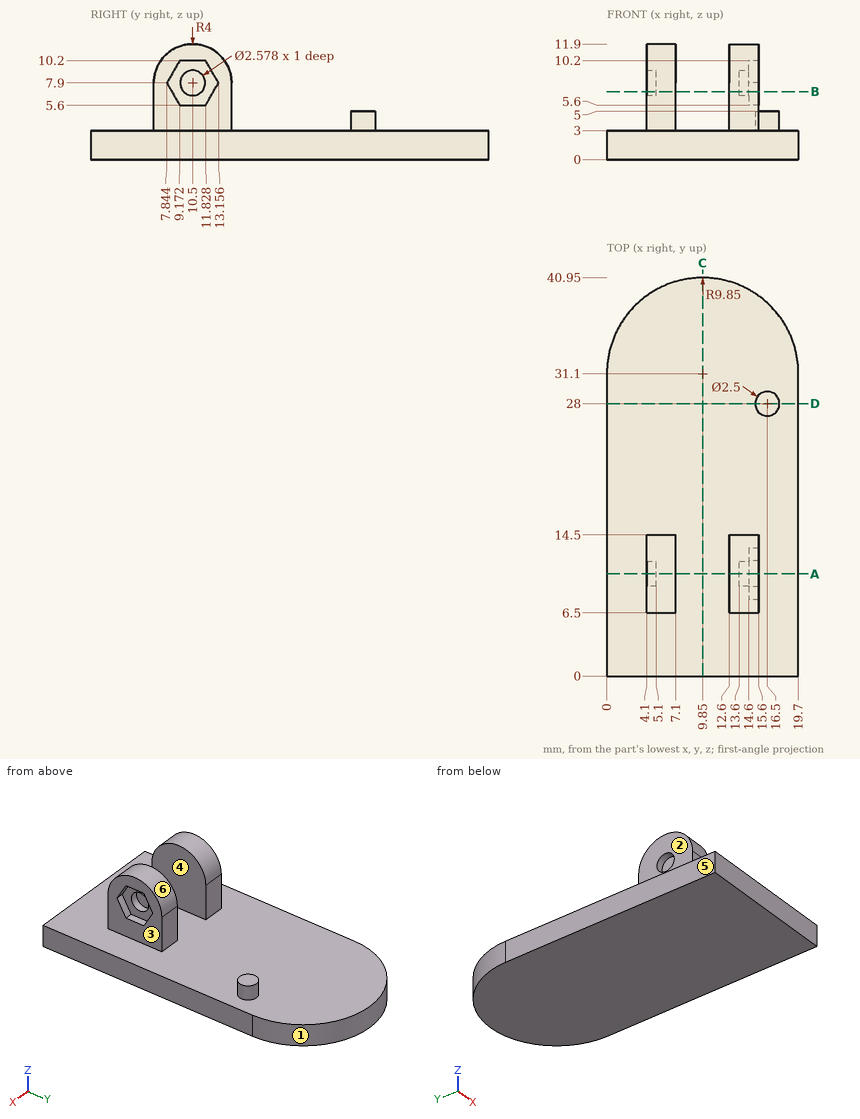
Print and shaded views of the part. All mm, measured from the part's lowest x, y and z. A direction names the side the tool comes from. Round coordinates to 2 decimals unless told otherwise and drop trailing zeros. Write each loop counter-clockwise with the first axis right and the second up, starting at its lowest first coordinate (ties: lowest second). Pieces come first, ordered by that corner, then holes.
(1) Slice it at A-A, the plane y = 10.5. Write the cut outline in (x, z).
(2) Probe line 1 along Z through (x, y) = (14.2, 10.5); line 2 along Y through (x, z) = (4.4, 7.9); line 3 along Z through (x, y) = (2, 26). List the from-to ranges inside material, lowest first.
(3) Mould opens along X. For the marked faces 4, 5 and 6 say: pulls with the +X half, pulls with the -X half, needs draft (parallel to the pull), parting line crosses it, or undercut.
(4) Slice it at D-D, the plane y = 28. Write the cut outline in (x, z), and give its area (3 significant figures).
(5) Drop flat-ended pins along their axis: P1, Ø4, axis at y = 9.5, z = 6, coming from the -X side; P2, Ø2.5, axis at y = 9.5, z = 6, coming from the +X side; P3, Ø1.5, axis at y = 10.5, z = 7.9, coming from the +X side. Give the stop position or say it passes through.
(6) Slice it at B-B, the plane z = 7. Write the cut outline in (x, y).
(7) 3-axis set-ups, long thin cutter, end or side, ignore diameter. For the marked faces 1, 2 and 3: which of +Z, -Z, +X, -X, +Y, -Y reach the whole face in a straight line?
(8) Slice it at C-C, the plane x = 9.85. Write the cut outline in (y, z).
From the geometry:
1. outline: (0, 0) - (19.7, 0) - (19.7, 3) - (15.6, 3) - (15.6, 5.6) - (14.6, 5.6) - (14.6, 6.61) - (13.6, 6.61) - (13.6, 9.19) - (14.6, 9.19) - (14.6, 10.2) - (15.6, 10.2) - (15.6, 11.9) - (12.6, 11.9) - (12.6, 3) - (7.1, 3) - (7.1, 11.9) - (4.1, 11.9) - (4.1, 9.19) - (5.1, 9.19) - (5.1, 6.61) - (4.1, 6.61) - (4.1, 3) - (0, 3) - close
2. line 1: z = 0 to 6.61, 9.19 to 11.9
2. line 2: y = 6.5 to 9.21, 11.79 to 14.5
2. line 3: z = 0 to 3
3. face 4: undercut
3. face 5: pulls with the -X half
3. face 6: needs draft
4. outline: (0, 0) - (19.7, 0) - (19.7, 3) - (17.75, 3) - (17.75, 5) - (15.25, 5) - (15.25, 3) - (0, 3) - close
4. area: 64.1 mm2
5. P1: stops at x = 4.1
5. P2: stops at x = 15.6
5. P3: stops at x = 13.6
6. outline: (4.1, 6.5) - (7.1, 6.5) - (7.1, 14.5) - (4.1, 14.5) - (4.1, 11.42) - (5.1, 11.42) - (5.1, 9.58) - (4.1, 9.58) - close; (12.6, 6.5) - (15.6, 6.5) - (15.6, 8.36) - (14.6, 8.36) - (14.6, 9.58) - (13.6, 9.58) - (13.6, 11.42) - (14.6, 11.42) - (14.6, 12.64) - (15.6, 12.64) - (15.6, 14.5) - (12.6, 14.5) - close
7. face 1: +Z, -Z, +Y
7. face 2: +Z, -X, +Y, -Y
7. face 3: +Z, +X, -Y
8. outline: (0, 0) - (40.95, 0) - (40.95, 3) - (0, 3) - close
